```python
from build123d import *

# Parameters (mm, degrees)
SKETCH1_W              = 95.89
SKETCH1_H              = 90.17
SUBSTRATE_DEPTH        = 1.6
SKETCH2_R              = 1.5
CUT_EXTRUDE2_DEPTH     = 10
SKETCH3_W              = 1.2
SKETCH3_H              = 1.2
SKETCH3_W_2            = 1
SKETCH3_H_2            = 1
CENTRE_ALIGNMENT_DEPTH = 10
SKETCH4_OUTSIDE_W      = 124.318
SKETCH4_OUTSIDE_H      = 118.598
CUT_EXTRUDE3_DEPTH     = 10


with BuildPart() as part:
    # Sketch1 → Substrate (new body)
    with BuildSketch(Plane(origin=(0, 0, 0), x_dir=(1, 0, 0), z_dir=(0, 1, 0))):
        Rectangle(SKETCH1_W, SKETCH1_H)
    extrude(amount=SUBSTRATE_DEPTH)

    # Sketch2 → Cut-Extrude2 (cut)
    with BuildSketch(Plane(origin=(0, 1.6, 0), x_dir=(1, 0, 0), z_dir=(0, 1, 0))):
        with Locations(Location((42.845, 36.085, 0), (0, 0, 270))):
            Circle(SKETCH2_R)
        with Locations(Location((42.845, -37.585, 0), (0, 0, 270))):
            Circle(SKETCH2_R)
        with Locations(Location((-42.945, -39.985, 0), (0, 0, 270))):
            Circle(SKETCH2_R)
        with Locations(Location((-42.945, 39.985, 0), (0, 0, 270))):
            Circle(SKETCH2_R)
    extrude(amount=-CUT_EXTRUDE2_DEPTH, mode=Mode.SUBTRACT)

    # Sketch3 → Centre Alignment (add)
    with BuildSketch(Plane(origin=(0, 1.6, 0), x_dir=(1, 0, 0), z_dir=(0, 1, 0))):
        Rectangle(SKETCH3_W, SKETCH3_H)
        Rectangle(SKETCH3_W_2, SKETCH3_H_2, mode=Mode.SUBTRACT)
    extrude(amount=CENTRE_ALIGNMENT_DEPTH)

    # Sketch4 outside → Cut-Extrude3 (cut)
    with BuildSketch(Plane(origin=(0, 1.6, 0), x_dir=(1, 0, 0), z_dir=(0, 1, 0))):
        Rectangle(SKETCH4_OUTSIDE_W, SKETCH4_OUTSIDE_H)
        with BuildLine():
            Line((-42.677096043, -44.977817588), (42.845, -42.685))
            ThreePointArc((42.845, -42.685), (46.451244584, -41.191244584), (47.945, -37.585))
            Line((47.945, -37.585), (47.945, 36.085))
            ThreePointArc((47.945, 36.085), (46.451244584, 39.691244584), (42.845, 41.185))
            Line((42.845, 41.185), (-42.502925272, 44.965418651))
            ThreePointArc((-42.502925272, 44.965418651), (-46.320620414, 43.673520953), (-47.945, 39.985))
            Line((-47.945, 39.985), (-47.945, -39.985))
            ThreePointArc((-47.945, -39.985), (-46.384511609, -43.614016381), (-42.677096043, -44.977817588))
        make_face(mode=Mode.SUBTRACT)
    extrude(amount=-CUT_EXTRUDE3_DEPTH, mode=Mode.SUBTRACT)


solid = part.part
```
Could you check a few things on this model? Use its own coordinates, in mm. Coordinates: 2 decimals unless noted, no trailing zeros. Order: outer loops, then holes, each group sorted by start corner. A loop starts at its lowest first (then second) coordinate and runs counter-clockwise, first axis right, second up. Notation, with made-up numbers: M 85.5,27.25 L 95.5,27.25 A10 cw 95.5,36.25 Z; hole C 82,35.5 d11. An arc over 180 degrees is marked long. Use a Markdown table: item, result. Add a question column.
Q1. If I drill on L1, parallel to Y at x = -13.5, z = 5; L2, parallel to Z at x = -35, y = 0.75, over which ranges is the centre line in solid material (lowest first)?
Q2. I'm going to push flat-ended pins straight in: pin 1 (0.5 mm diameter, centred on y = 7.5, z = 0, fed in from -X); pin 2 (4 mm diameter, centred on x = 42.845, z = -36.085, fed in from +Y); pin 3 (0.5 mm diameter, centred on x = 0, y = 5.5, fed in from -Z). Where does each tip first touch, or does it pass through?
Q3. I want a section at C-C on x = 36. List the corners of the cut face in (y, z) for me, then the cut area to 3 significant figures.
Q4. I want a section at A-A on y = 10.25. List the corners of the cut face in (x, z) for me.
Q5. I want a section at B-B on z = 19. List the corners of the cut face in (x, y) for me (3 decimals).
Q6. We'd pull the mould along Z, two halves only. Please class faces 1 (the cylindrical face through (-43.52, 0.81, 41.37)), 2 (the cylindrical face through (46.49, 0.81, -39.65)), 3 (the cylindrical face through (46.41, 0.81, 41.23)): pulls with the +Z half, pulls with the -Z half, needs draft (parallel to the pull), parting line crosses it, or undercut.
Checked values:
| question | item | result |
|---|---|---|
| 1 | L1 | 0 to 1.6 |
| 1 | L2 | -44.63 to 44.77 |
| 2 | pin 1 | x = -0.6 |
| 2 | pin 2 | y = 1.6 |
| 2 | pin 3 | z = -0.6 |
| 3 | outline | M 0,-41.49 L 1.6,-41.49 L 1.6,42.87 L 0,42.87 Z |
| 3 | area | 135 mm² |
| 4 | outline | M -0.6,-0.6 L 0.6,-0.6 L 0.6,0.6 L -0.6,0.6 Z; hole M -0.5,-0.5 L 0.5,-0.5 L 0.5,0.5 L -0.5,0.5 Z |
| 5 | outline | M -47.945,0 L 47.945,0 L 47.945,1.6 L -47.945,1.6 Z |
| 6 | face 1 | undercut |
| 6 | face 2 | pulls with the -Z half |
| 6 | face 3 | pulls with the +Z half |
